```python
from build123d import *

# Parameters (mm, degrees)
ESQUISSE2_W                  = 16
ESQUISSE2_H                  = 9.5
BOSS_EXTRU_1_DEPTH           = 2
ESQUISSE5_W                  = 16
ESQUISSE5_H                  = 2
BOSS_EXTRU_2_DEPTH           = 15
ENL_V_MAT_EXTRU_1_DEPTH      = 1
ENL_V_MAT_EXTRU_1_DEPTH_BACK = 12.5
ESQUISSE7_W                  = 2
ESQUISSE7_H                  = 15
BOSS_EXTRU_3_DEPTH           = 14
BOSS_EXTRU_4_DEPTH           = 1
ENL_V_MAT_EXTRU_2_REACH      = 13.5
ESQUISSE9_R                  = 3
ENL_V_MAT_EXTRU_3_REACH      = 4
ESQUISSE11_R                 = 1.5
CHANFREIN1_SIZE              = 1
CHANFREIN1_SIZE2             = 1.732050808


with BuildPart() as part:
    # Esquisse2 → Boss.-Extru.1 (new body)
    with BuildSketch(Plane(origin=(0, 0, 0), x_dir=(1, 0, 0), z_dir=(0, 1, 0))):
        with Locations((0, 4.75)):
            Rectangle(ESQUISSE2_W, ESQUISSE2_H)
    extrude(amount=BOSS_EXTRU_1_DEPTH)

    # Esquisse5 → Boss.-Extru.2 (add)
    with BuildSketch(Plane.XZ):
        with Locations((0, -10.5)):
            Rectangle(ESQUISSE5_W, ESQUISSE5_H)
    extrude(amount=-BOSS_EXTRU_2_DEPTH)

    # Esquisse6 → Enlèv. mat.-Extru.1 (cut, two sides)
    with BuildSketch(Plane(origin=(0, 0, -11.5), x_dir=(-1, 0, 0), z_dir=(0, 0, -1))) as enl_v_mat_extru_1_sk:
        Polygon((-48.758415637, 38.562223804), (-5, 15), (8, 8), (51.758415637, -15.562223804), (98.882863246, 71.954607469), (-1.633968028, 126.079055078), align=None)
    extrude(amount=ENL_V_MAT_EXTRU_1_DEPTH, mode=Mode.SUBTRACT)
    extrude(enl_v_mat_extru_1_sk.sketch, amount=-ENL_V_MAT_EXTRU_1_DEPTH_BACK, mode=Mode.SUBTRACT)

    # Esquisse7 → Boss.-Extru.3 (add)
    with BuildSketch(Plane(origin=(8, 0, 0), x_dir=(0, 0, -1), z_dir=(1, 0, 0))):
        with Locations((10.5, 7.5)):
            Rectangle(ESQUISSE7_W, ESQUISSE7_H)
    extrude(amount=BOSS_EXTRU_3_DEPTH)

    # Esquisse8 → Boss.-Extru.4 (add)
    with BuildSketch(Plane.XY.offset(-9.5)):
        Polygon((-8, 2), (-8, 4), (3, 9.923076923), (3, 2), align=None)
    extrude(amount=BOSS_EXTRU_4_DEPTH)

    # Esquisse9 → Enlèv. mat.-Extru.2 (cut, up to next)
    with BuildSketch(Plane(origin=(0, 0, -11.5), x_dir=(-1, 0, 0), z_dir=(0, 0, -1)), mode=Mode.PRIVATE) as enl_v_mat_extru_2_sk1:
        with Locations((-14.5, 7.5)):
            Circle(ESQUISSE9_R)
    enl_v_mat_extru_2_tool1 = extrude(enl_v_mat_extru_2_sk1.sketch, amount=-ENL_V_MAT_EXTRU_2_REACH, mode=Mode.PRIVATE) & part.part
    add(enl_v_mat_extru_2_tool1.solids().sort_by_distance((14.5, 7.5, -11.5))[0], mode=Mode.SUBTRACT)

    # Symétrie1: part across plane


with BuildPart() as part_1:
    add(part.part)
    add(part.part.mirror(Plane(origin=(-8, 2, 0), x_dir=(1, 0, 0), z_dir=(0, 0, -1))))

    # Esquisse11 → Enlèv. mat.-Extru.3 (cut, up to next)
    with BuildSketch(Plane(origin=(0, 2, 0), x_dir=(1, 0, 0), z_dir=(0, 1, 0)), mode=Mode.PRIVATE) as enl_v_mat_extru_3_sk1:
        with Locations((-4, 0)):
            Circle(ESQUISSE11_R)
    enl_v_mat_extru_3_tool1 = extrude(enl_v_mat_extru_3_sk1.sketch, amount=-ENL_V_MAT_EXTRU_3_REACH, mode=Mode.PRIVATE) & part_1.part
    add(enl_v_mat_extru_3_tool1.solids().sort_by_distance((-4, 2, 0))[0], mode=Mode.SUBTRACT)
    # Esquisse11 → Enlèv. mat.-Extru.3 (cut, up to next)
    with BuildSketch(Plane(origin=(0, 2, 0), x_dir=(1, 0, 0), z_dir=(0, 1, 0)), mode=Mode.PRIVATE) as enl_v_mat_extru_3_sk2:
        with Locations((4, 0)):
            Circle(ESQUISSE11_R)
    enl_v_mat_extru_3_tool2 = extrude(enl_v_mat_extru_3_sk2.sketch, amount=-ENL_V_MAT_EXTRU_3_REACH, mode=Mode.PRIVATE) & part_1.part
    add(enl_v_mat_extru_3_tool2.solids().sort_by_distance((4, 2, 0))[0], mode=Mode.SUBTRACT)

    # Chanfrein1
    chanfrein1_edges = [part_1.edges().sort_by_distance(p)[0] for p in [
        (-5.5, 2, 0),
        (2.5, 2, 0),
    ]]
    chanfrein1_side = [part_1.faces().sort_by_distance(p)[0] for p in [
        (0.205328971, 2, 0),
    ]]
    chamfer(chanfrein1_edges, length=CHANFREIN1_SIZE, length2=CHANFREIN1_SIZE2, reference=chanfrein1_side[0])


solid = part_1.part
```
Geometry check sheet. Reference: the model listing, model coordinates, mm. A direction names the side the tool comes from. Give positions to 0.01 mm unless a question says otherwise; leave off trailing zeros. Order: outer loops, then holes, each group sorted by start corner. A loop starts at its lowest first (then second) coordinate and runs counter-clockwise, first axis right, second up.
1. Access from +Z, -Z, +X, -X, +Y, -Y to the whole of each face (thin tool, end or side, straight path). Record for faces 1 (the face through (-2.58, 6.92, 9.01)), 2 (the face through (22, 8, -10)).
2. Section check A-A, the plane x = 14.5. Enter the section's corners in (y, z), and give its area (3 significant figures).
3. Section check B-B, the plane y = 2.5. Enter the section's corners in (x, z), and give its area (3 significant figures).
4. Release check for a two-part mould opening along Z. For faces 3 (the face through (3, 6, -9)), 4 (the face through (-1.41, 11.55, 10.51)), 5 (the face through (7, 7, 11.5)) record: pulls with the +Z half, pulls with the -Z half, needs draft (parallel to the pull), parting line crosses it, or undercut.
5. Section check C-C, the plane x = 18. Enter the section's corners in (y, z), and give its area (3 significant figures).
6. Gauge pin test, flat ends, axial feed: pin 1 Ø5 at (x, z) = (-1.5, -0.5) entering from +Y; pin 2 Ø8 at (y, z) = (11, 3.5) entering from +X; pin 3 Ø2 at (y, z) = (0.5, -4.5) entering from +X; pin 4 Ø0.8 at (y, z) = (7.5, -9) entering from +X. Record the tip position at first contact, or that the pin passes through.
7. Thickness scan on L1, parallel to X at y = 0.2, z = 0; L2, parallel to Z at x = 9, y = 14.25; L3, parallel to Z at x = -2.25, y = 2.75. Record the ranges inside material, lowest first.
8. Section check D-D, the plane z = 0. Enter the section's corners in (x, y), and give its area (3 significant figures).
Values follow:
1. face 1: -X, +Y
1. face 2: +Z, -Z, +X, +Y, -Y
2. outline: (0, -11.5) - (4.5, -11.5) - (4.5, -9.5) - (0, -9.5) - close; (0, 9.5) - (4.5, 9.5) - (4.5, 11.5) - (0, 11.5) - close; (10.5, -11.5) - (15, -11.5) - (15, -9.5) - (10.5, -9.5) - close; (10.5, 9.5) - (15, 9.5) - (15, 11.5) - (10.5, 11.5) - close
2. area: 36.0 mm2
3. outline: (-8, -11.5) - (22, -11.5) - (22, -9.5) - (3, -9.5) - (3, -8.5) - (-8, -8.5) - close; (-8, 8.5) - (3, 8.5) - (3, 9.5) - (22, 9.5) - (22, 11.5) - (-8, 11.5) - close
3. area: 142 mm2
4. face 3: undercut
4. face 4: needs draft
4. face 5: pulls with the +Z half
5. outline: (0, -11.5) - (15, -11.5) - (15, -9.5) - (0, -9.5) - close; (0, 9.5) - (15, 9.5) - (15, 11.5) - (0, 11.5) - close
5. area: 60.0 mm2
6. pin 1: stops at y = 2
6. pin 2: passes through
6. pin 3: stops at x = 8
6. pin 4: stops at x = 3
7. L1: x = -8 to -5.5, -2.5 to 2.5, 5.5 to 8
7. L2: z = -11.5 to -9.5, 9.5 to 11.5
7. L3: z = -11.5 to -8.5, 8.5 to 11.5
8. outline: (-8, 0) - (-5.5, 0) - (-5.5, 0.27) - (-6.5, 2) - (-8, 2) - close; (-2.5, 0) - (2.5, 0) - (2.5, 0.27) - (1.5, 2) - (-1.5, 2) - (-2.5, 0.27) - close; (5.5, 0) - (8, 0) - (8, 2) - (6.5, 2) - (5.5, 0.27) - close
8. area: 16.5 mm2
